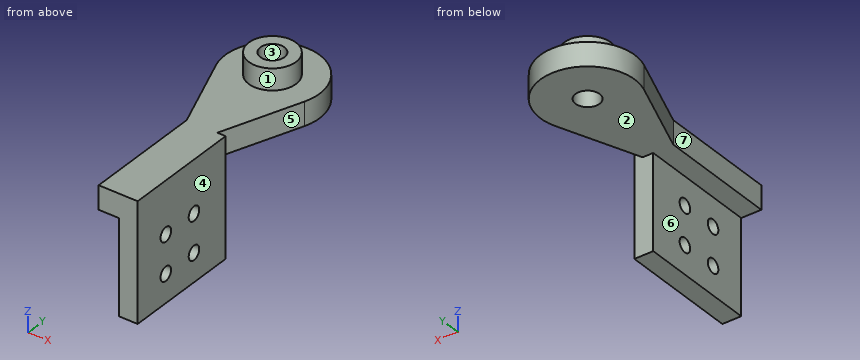
```python
from build123d import *

# Parameters (mm, degrees)
SKETCH_1_R          = 1.25
EXTRUDE_1_DEPTH     = 5
SKETCH_2_W          = 5
SKETCH_2_H          = 25
EXTRUDE_2_DEPTH     = 4
SKETCH_3_W          = 4
SKETCH_3_H          = 25
EXTRUDE_3_DEPTH     = 20
SKETCH_4_R          = 1.5
CUT_EXTRUDE_1_DEPTH = 20
EXTRUDE_START       = -5
SKETCH_7_R          = 1.25
EXTRUDE_4_DEPTH     = 5
SKETCH_8_R          = 1.5
SKETCH_8_R_2        = 4
EXTRUDE_5_DEPTH     = 5
EXTRUDE_START_2     = 4
SKETCH_14_W         = 25
SKETCH_14_H         = 25
SKETCH_14_R         = 1.5
EXTRUDE_9_DEPTH     = 4
SKETCH_15_W         = 4
SKETCH_15_H         = 25
CUT_EXTRUDE_2_DEPTH = 100
SKETCH_16_R         = 10.000418411
SKETCH_16_R_2       = 2.55
EXTRUDE_10_DEPTH    = 5
EXTRUDE_START_3     = 4.5
SKETCH_18_R         = 5
SKETCH_18_R_2       = 2.55
EXTRUDE_11_DEPTH    = 4.5
SKETCH_19_W         = 25
SKETCH_19_H         = 25
SKETCH_19_R         = 1.5
EXTRUDE_12_DEPTH    = 4
SKETCH_20_W         = 25
SKETCH_20_H         = 25
CUT_EXTRUDE_3_DEPTH = 4
SKETCH_21_W         = 1.749900533
SKETCH_21_H         = 25
EXTRUDE_13_DEPTH    = 20
CUT_EXTRUDE_START   = -20
SKETCH_22_R         = 1.5
CUT_EXTRUDE_4_DEPTH = 20
SKETCH_23_W         = 25
SKETCH_23_H         = 25
CUT_EXTRUDE_5_DEPTH = 4
SKETCH_24_W         = 1.749900533
SKETCH_24_H         = 25
EXTRUDE_14_DEPTH    = 5


with BuildPart() as part:
    # 草图1 → 凸台-拉伸1 (new body)
    with BuildSketch(Plane.XY):
        Polygon((-3.581151343, -8.027992706), (-3.581151343, -12.611885422), (2.918848657, -12.611885422), (2.918848657, -6.641886627), (2.918848657, 12.388114578), (-3.581151343, 12.388114578), align=None)
        with Locations((-0.081151343, 8.237522913)):
            Circle(SKETCH_1_R, mode=Mode.SUBTRACT)
        with Locations((-0.081151343, 2.787522913)):
            Circle(SKETCH_1_R, mode=Mode.SUBTRACT)
        with Locations((-0.081151343, -2.662477087)):
            Circle(SKETCH_1_R, mode=Mode.SUBTRACT)
        with Locations((-0.000846901, -8.111885422)):
            Circle(SKETCH_1_R, mode=Mode.SUBTRACT)
    extrude(amount=EXTRUDE_1_DEPTH)

    # 草图2 → 凸台-拉伸2 (add)
    with BuildSketch(Plane.ZY.offset(3.581151343)):
        with Locations((2.5, -0.111885422)):
            Rectangle(SKETCH_2_W, SKETCH_2_H)
    extrude(amount=EXTRUDE_2_DEPTH)

    # 草图3 → 凸台-拉伸3 (add)
    with BuildSketch(Plane(origin=(0, 0, 0), x_dir=(-1, 0, 0), z_dir=(0, 0, -1))):
        with Locations((5.581151343, -0.111885422)):
            Rectangle(SKETCH_3_W, SKETCH_3_H)
    extrude(amount=EXTRUDE_3_DEPTH)

    # 草图4 → 切除-拉伸1 (cut)
    with BuildSketch(Plane(origin=(-3.581151343, 0, 0), x_dir=(0, 0, -1), z_dir=(1, 0, 0))):
        with Locations(Location((6, 3.388114578, 0), (0, 0, 90))):
            Circle(SKETCH_4_R)
        with Locations(Location((14, 3.388114578, 0), (0, 0, 180))):
            Circle(SKETCH_4_R)
        with Locations(Location((14, -4.611885422, 0), (0, 0, 90))):
            Circle(SKETCH_4_R)
        with Locations(Location((6, -4.611885422, 0), (0, 0, 180))):
            Circle(SKETCH_4_R)
    extrude(amount=-CUT_EXTRUDE_1_DEPTH, mode=Mode.SUBTRACT)

    # 草图7 → 凸台-拉伸4 (add)
    with BuildSketch(Plane.XY.offset(5).offset(EXTRUDE_START)):
        with Locations((-0.081151343, 8.237522913)):
            Circle(SKETCH_7_R)
        with Locations((-0.081151343, 2.787522913)):
            Circle(SKETCH_7_R)
        with Locations((-0.081151343, -2.662477087)):
            Circle(SKETCH_7_R)
        with Locations((-0.000846901, -8.111885422)):
            Circle(SKETCH_7_R)
    extrude(amount=EXTRUDE_4_DEPTH)

    # 草图8 → 凸台-拉伸5 (add)
    with BuildSketch(Plane.XY.offset(5)):
        with BuildLine():
            ThreePointArc((9.045368421, 28.911309576), (-0.331303735, 42.388418969), (-9.707833242, 28.911210329))
            Line((-9.707833242, 28.911210329), (-3.581151343, 12.388114578))
            Line((-3.581151343, 12.388114578), (2.918848657, 12.388114578))
            Line((2.918848657, 12.388114578), (9.045368421, 28.911309576))
        make_face()
        with Locations((-0.33125081, 25.388000558)):
            Circle(SKETCH_8_R, mode=Mode.SUBTRACT)
        with Locations((-7.33125081, 32.388000558)):
            Circle(SKETCH_8_R, mode=Mode.SUBTRACT)
        with Locations((-0.33125081, 32.388000558)):
            Circle(SKETCH_8_R_2, mode=Mode.SUBTRACT)
        with Locations((-0.33125081, 39.388000558)):
            Circle(SKETCH_8_R, mode=Mode.SUBTRACT)
        with Locations((6.668848657, 32.388114578)):
            Circle(SKETCH_8_R, mode=Mode.SUBTRACT)
    extrude(amount=-EXTRUDE_5_DEPTH)

    # 草图14 → 凸台-拉伸9 (add)
    with BuildSketch(Plane(origin=(2.918848657, 0, 0), x_dir=(0, 0, -1), z_dir=(1, 0, 0)).offset(EXTRUDE_START_2)):
        with Locations((7.5, -0.111885422)):
            Rectangle(SKETCH_14_W, SKETCH_14_H)
        with Locations(Location((6, 3.388114578, 0), (0, 0, 90))):
            Circle(SKETCH_14_R, mode=Mode.SUBTRACT)
        with Locations(Location((14, 3.388114578, 0), (0, 0, 180))):
            Circle(SKETCH_14_R, mode=Mode.SUBTRACT)
        with Locations(Location((14, -4.611885422, 0), (0, 0, 90))):
            Circle(SKETCH_14_R, mode=Mode.SUBTRACT)
        with Locations(Location((6, -4.611885422, 0), (0, 0, 180))):
            Circle(SKETCH_14_R, mode=Mode.SUBTRACT)
    extrude(amount=-EXTRUDE_9_DEPTH)

    # 草图15 → 切除-拉伸2 (cut)
    with BuildSketch(Plane(origin=(0, 0, -20), x_dir=(-1, 0, 0), z_dir=(0, 0, -1))):
        with Locations((5.581151343, -0.111885422)):
            Rectangle(SKETCH_15_W, SKETCH_15_H)
    extrude(amount=-CUT_EXTRUDE_2_DEPTH, mode=Mode.SUBTRACT)

    # 草图16 → 凸台-拉伸10 (add)
    with BuildSketch(Plane.XY.offset(5)):
        with Locations((-0.33125081, 32.388000558)):
            Circle(SKETCH_16_R)
        with Locations((-0.33125081, 32.388000558)):
            Circle(SKETCH_16_R_2, mode=Mode.SUBTRACT)
    extrude(amount=-EXTRUDE_10_DEPTH)

    # 草图18 → 凸台-拉伸11 (add)
    with BuildSketch(Plane.XY.offset(5).offset(EXTRUDE_START_3)):
        with Locations(Location((-0.33125081, 32.388000558, 0), (0, 0, 180))):
            Circle(SKETCH_18_R)
        with Locations((-0.33125081, 32.388000558)):
            Circle(SKETCH_18_R_2, mode=Mode.SUBTRACT)
    extrude(amount=-EXTRUDE_11_DEPTH)

    # 草图19 → 凸台-拉伸12 (add)
    with BuildSketch(Plane.ZY.offset(3.581151343)):
        with Locations((-7.5, -0.111885422)):
            Rectangle(SKETCH_19_W, SKETCH_19_H)
        with Locations(Location((-14, 3.388114578, 0), (0, 0, 90))):
            Circle(SKETCH_19_R, mode=Mode.SUBTRACT)
        with Locations(Location((-6, 3.388114578, 0), (0, 0, 90))):
            Circle(SKETCH_19_R, mode=Mode.SUBTRACT)
        with Locations(Location((-14, -4.611885422, 0), (0, 0, 90))):
            Circle(SKETCH_19_R, mode=Mode.SUBTRACT)
        with Locations(Location((-6, -4.611885422, 0), (0, 0, 90))):
            Circle(SKETCH_19_R, mode=Mode.SUBTRACT)
    extrude(amount=EXTRUDE_12_DEPTH)

    # 草图20 → 切除-拉伸3 (cut)
    with BuildSketch(Plane(origin=(6.918848657, 0, 0), x_dir=(0, 0, -1), z_dir=(1, 0, 0))):
        with Locations((7.5, -0.111885422)):
            Rectangle(SKETCH_20_W, SKETCH_20_H)
    extrude(amount=-CUT_EXTRUDE_3_DEPTH, mode=Mode.SUBTRACT)

    # 草图21 → 凸台-拉伸13 (add)
    with BuildSketch(Plane(origin=(0, 0, 0), x_dir=(-1, 0, 0), z_dir=(0, 0, -1))):
        Polygon((-0.66874919, -12.611885422), (-0.66874919, 5.526794347), (-0.66874919, 12.388114578), (-2.918848657, 12.388114578), (-2.918848657, -12.611885422), align=None)
        with Locations((-3.793798924, -0.111885422)):
            Rectangle(SKETCH_21_W, SKETCH_21_H)
    extrude(amount=EXTRUDE_13_DEPTH)

    # 草图22 → 切除-拉伸4 (cut)
    with BuildSketch(Plane.ZY.offset(7.581151343).offset(CUT_EXTRUDE_START)):
        with Locations((-14, 3.388114578)):
            Circle(SKETCH_22_R)
        with Locations((-6, 3.388114578)):
            Circle(SKETCH_22_R)
        with Locations((-14, -4.611885422)):
            Circle(SKETCH_22_R)
        with Locations((-6, -4.611885422)):
            Circle(SKETCH_22_R)
    extrude(amount=CUT_EXTRUDE_4_DEPTH, mode=Mode.SUBTRACT)

    # 草图23 → 切除-拉伸5 (cut)
    with BuildSketch(Plane.ZY.offset(7.581151343)):
        with Locations((-7.5, -0.111885422)):
            Rectangle(SKETCH_23_W, SKETCH_23_H)
    extrude(amount=-CUT_EXTRUDE_5_DEPTH, mode=Mode.SUBTRACT)

    # 草图24 → 凸台-拉伸14 (add)
    with BuildSketch(Plane.XY):
        with Locations((3.793798924, -0.111885422)):
            Rectangle(SKETCH_24_W, SKETCH_24_H)
    extrude(amount=EXTRUDE_14_DEPTH)


solid = part.part
```
The model under review builds one solid part; all positions refer to its coordinate system, in mm. Face numbers are marked on the shaded views. A direction names the side the tool comes from. Coordinates: 2 decimals unless noted, no trailing zeros. Write each loop counter-clockwise with the first axis right and the second up, starting at its lowest first coordinate (ties: lowest second). Pieces come first, ordered by that corner, then holes. Notation, with made-up numbers: (-17, 20.25) -> (24, 20.25) arc R17 cw to (24, 50.25) -> close; hole circle Ø4 at (-20, 64.25). An arc over 180 degrees is marked (long way). One line per item, written item: value. Start each with the question number.
Q1. For the marked faces 4, 5, 6 and 7, list the 3-axis set-ups (+Z, -Z, +X, -X, +Y, -Y) from which the entire face can be reached by the end or side of a thin tool; tool diameter is ignored.
Q2. Add section C-C, the plane y = -7.5. Give the boundary of the cut face in (x, z), then the cut area to 3 significant figures.
Q3. Add section A-A, the plane z = -6. Give the boundary of the cut face in (x, y).
Q4. The part is to be moulded in two halves that separate along Y. For the marked faces 1, 2 and 3, say which applies: +Y half, -Y half, draft (parallel to the pull), parting line (faces both ways), or undercut.
Q5. To check wall thickness, follow probe 1 along Y at (x, z) = (1.55, -6); probe 2 along Z at (x, y) = (0.25, 7); probe 3 along X at (y, z) = (11, -13). State the ranges of each line that lie inside material, in increasing order.
Q6. Clearance check with flat-ended pins moving along their axes: P1, Ø16, axis at y = 4.5, z = -7.5, coming from the -X side; P2, Ø7.5, axis at y = 0.5, z = -3.5, coming from the +X side; P3, Ø4, axis at x = 4, z = -0.5, coming from the +Y side; P4, Ø2.5, axis at y = 3.39, z = -14, coming from the -X side. State where each tip first meets the part, or that it passes through.
Q7. Add section D-D, the plane x = 5.5. Give the boundary of the cut face in (y, z).
Q8. Add section B-B, the plane x = -1.25. Give the boundary of the cut face in (y, z).
Response:
1. face 4: +Z, -Z, +X, -Y
1. face 5: +Z, -Z, +X
1. face 6: -Z, -X, +Y, -Y
1. face 7: +Z, -Z, -X, -Y
2. outline: (-3.58, 0) -> (0.67, 0) -> (0.67, -20) -> (4.67, -20) -> (4.67, 5) -> (-3.58, 5) -> close
2. area: 121 mm²
3. outline: (0.67, -12.61) -> (4.67, -12.61) -> (4.67, -6.11) -> (0.67, -6.11) -> close; (0.67, -3.11) -> (4.67, -3.11) -> (4.67, 1.89) -> (0.67, 1.89) -> close; (0.67, 4.89) -> (4.67, 4.89) -> (4.67, 12.39) -> (0.67, 12.39) -> close
4. face 1: parting line
4. face 2: draft
4. face 3: undercut
5. probe 1: -12.61 to -6.11, -3.11 to 1.89, 4.89 to 12.39
5. probe 2: 0 to 5
5. probe 3: 0.67 to 4.67
6. P1: x = -3.58
6. P2: x = 4.67
6. P3: y = 42.1
6. P4: through
7. outline: (19.35, 0) -> (40.51, 0) -> (40.51, 5) -> (19.35, 5) -> close
8. outline: (-12.61, 0) -> (30.01, 0) -> (30.01, 9.5) -> (27.47, 9.5) -> (27.47, 5) -> (-12.61, 5) -> close; (34.77, 0) -> (42.35, 0) -> (42.35, 5) -> (37.3, 5) -> (37.3, 9.5) -> (34.77, 9.5) -> close
